```python
from build123d import *

# Parameters (mm, degrees)
BOSS_EXTRUDE1_DEPTH             = 3
BOSS_EXTRUDE2_START             = -6
BOSS_EXTRUDE2_DEPTH             = 6
TAP_DRILL_FOR_M3X0_5_TAP1_D     = 2.5
TAP_DRILL_FOR_M3X0_5_TAP1_DEPTH = 10
TAP_DRILL_FOR_M3X0_5_TAP1_TIP   = 0.751075774
M3_CLEARANCE_HOLE1_D            = 3.4
M3_CLEARANCE_HOLE1_DEPTH        = 10
M3_CLEARANCE_HOLE1_TIP          = 1.021463052
M3_CLEARANCE_HOLE2_D            = 3.4
M3_CLEARANCE_HOLE2_DEPTH        = 10
M3_CLEARANCE_HOLE2_TIP          = 1.021463052
BOSS_EXTRUDE3_START             = 2.5
SKETCH9_R                       = 1.7
BOSS_EXTRUDE3_DEPTH             = 2.5
TAP_DRILL_FOR_M3X0_5_TAP2_D     = 2.5
TAP_DRILL_FOR_M3X0_5_TAP2_DEPTH = 10
TAP_DRILL_FOR_M3X0_5_TAP2_TIP   = 0.751075774
SKETCH8_W                       = 1.5
SKETCH8_H                       = 3.5
CUT_EXTRUDE1_DEPTH              = 15
FILLET3_R                       = 3
FILLET4_R                       = 10


# Some blends are built 0.0001 mm under size
with BuildPart() as part:
    # Sketch1 → Boss-Extrude1 (new body)
    with BuildSketch(Plane.XY):
        with BuildLine():
            Line((-5.729559867, 10.267386408), (-20.186344056, -8.782393513))
            ThreePointArc((-20.186344056, -8.782393513), (-19.418100816, -14.386838385), (-13.813655944, -13.618595145))
            Line((-13.813655944, -13.618595145), (0, 4.583731333))
            Line((0, 4.583731333), (13.813655944, -13.618595145))
            ThreePointArc((13.813655944, -13.618595145), (19.418100816, -14.386838385), (20.186344056, -8.782393513))
            Line((20.186344056, -8.782393513), (5.729559867, 10.267386408))
            Line((5.729559867, 10.267386408), (19.254422206, 19.495329447))
            ThreePointArc((19.254422206, 19.495329447), (20.822087446, 23.979186794), (17, 26.799505671))
            Line((17, 26.799505671), (7, 26.799505671))
            Line((7, 26.799505671), (7, 66.799505671))
            ThreePointArc((7, 66.799505671), (0, 73.799505671), (-7, 66.799505671))
            Line((-7, 66.799505671), (-7, 26.799505671))
            Line((-7, 26.799505671), (-17, 26.799505671))
            ThreePointArc((-17, 26.799505671), (-20.822087446, 23.979186794), (-19.254422206, 19.495329447))
            Line((-19.254422206, 19.495329447), (-5.729559867, 10.267386408))
        make_face()
    extrude(amount=BOSS_EXTRUDE1_DEPTH)

    # Sketch1<3> → Boss-Extrude2 (add)
    with BuildSketch(Plane.XY.offset(BOSS_EXTRUDE2_START)):
        with BuildLine():
            ThreePointArc((-21, 22.799505671), (-20.536784473, 20.931042241), (-19.254422206, 19.495329447))
            ThreePointArc((-19.254422206, 19.495329447), (-15.13153657, 19.262721197), (-13, 22.799505671))
            ThreePointArc((-13, 22.799505671), (-13.463215527, 24.667969101), (-14.745577794, 26.103681895))
            ThreePointArc((-14.745577794, 26.103681895), (-15.820318877, 26.621593117), (-17, 26.799505671))
            ThreePointArc((-17, 26.799505671), (-19.828427125, 25.627932795), (-21, 22.799505671))
        make_face()
        with BuildLine():
            ThreePointArc((14.745577794, 26.103681895), (13.695823776, 20.545083465), (19.254422206, 19.495329447))
            ThreePointArc((19.254422206, 19.495329447), (20.536784473, 20.931042241), (21, 22.799505671))
            ThreePointArc((21, 22.799505671), (19.828427125, 25.627932795), (17, 26.799505671))
            ThreePointArc((17, 26.799505671), (15.820318877, 26.621593117), (14.745577794, 26.103681895))
        make_face()
        with BuildLine():
            ThreePointArc((20.186344056, -8.782393513), (14.581899184, -8.014150273), (13.813655944, -13.618595145))
            ThreePointArc((13.813655944, -13.618595145), (15.221293063, -14.783258853), (17, -15.200494329))
            ThreePointArc((17, -15.200494329), (19.828427125, -14.028921454), (21, -11.200494329))
            ThreePointArc((21, -11.200494329), (20.791132827, -9.924832976), (20.186344056, -8.782393513))
        make_face()
        with BuildLine():
            ThreePointArc((-17, -15.200494329), (-15.221293063, -14.783258853), (-13.813655944, -13.618595145))
            ThreePointArc((-13.813655944, -13.618595145), (-13.208867173, -12.476155682), (-13, -11.200494329))
            ThreePointArc((-13, -11.200494329), (-15.724338647, -7.409361502), (-20.186344056, -8.782393513))
            ThreePointArc((-20.186344056, -8.782393513), (-20.791132827, -9.924832976), (-21, -11.200494329))
            ThreePointArc((-21, -11.200494329), (-19.828427125, -14.028921454), (-17, -15.200494329))
        make_face()
    extrude(amount=BOSS_EXTRUDE2_DEPTH)

    # Tap Drill for M3x0.5 Tap1
    with Locations(Plane(origin=(0, 0, -6), x_dir=(-1, 0, 0), z_dir=(0, 0, -1))):
        with Locations((17, 22.799505671), (-17, 22.799505671)):
            Hole(TAP_DRILL_FOR_M3X0_5_TAP1_D / 2, depth=TAP_DRILL_FOR_M3X0_5_TAP1_DEPTH)
            with Locations((0, 0, -(TAP_DRILL_FOR_M3X0_5_TAP1_DEPTH + TAP_DRILL_FOR_M3X0_5_TAP1_TIP / 2))):  # 118° drill point
                Cone(0, TAP_DRILL_FOR_M3X0_5_TAP1_D / 2, TAP_DRILL_FOR_M3X0_5_TAP1_TIP, mode=Mode.SUBTRACT)

    # M3 Clearance Hole1
    with Locations(Plane(origin=(0, 0, -6), x_dir=(-1, 0, 0), z_dir=(0, 0, -1))):
        with Locations((-17, -11.200494329), (17, -11.200494329)):
            Hole(M3_CLEARANCE_HOLE1_D / 2, depth=M3_CLEARANCE_HOLE1_DEPTH)
            with Locations((0, 0, -(M3_CLEARANCE_HOLE1_DEPTH + M3_CLEARANCE_HOLE1_TIP / 2))):  # 118° drill point
                Cone(0, M3_CLEARANCE_HOLE1_D / 2, M3_CLEARANCE_HOLE1_TIP, mode=Mode.SUBTRACT)

    # M3 Clearance Hole2
    with Locations(Plane.XY.offset(3)):
        with Locations((0, 11.200494329)):
            Hole(M3_CLEARANCE_HOLE2_D / 2, depth=M3_CLEARANCE_HOLE2_DEPTH)
            with Locations((0, 0, -(M3_CLEARANCE_HOLE2_DEPTH + M3_CLEARANCE_HOLE2_TIP / 2))):  # 118° drill point
                Cone(0, M3_CLEARANCE_HOLE2_D / 2, M3_CLEARANCE_HOLE2_TIP, mode=Mode.SUBTRACT)

    # Sketch9 → Boss-Extrude3 (add)
    with BuildSketch(Plane(origin=(0, 0, 0), x_dir=(-1, 0, 0), z_dir=(0, 0, -1)).offset(BOSS_EXTRUDE3_START)):
        with BuildLine():
            Line((7, 66.799505671), (4.365625, 66.799505671))
            Line((4.365625, 66.799505671), (4.365625, 26.799505671))
            Line((4.365625, 26.799505671), (-4.365625, 26.799505671))
            Line((-4.365625, 26.799505671), (-4.365625, 66.799505671))
            Line((-4.365625, 66.799505671), (-7, 66.799505671))
            Line((-7, 66.799505671), (-7, 26.799505671))
            Line((-7, 26.799505671), (-17, 26.799505671))
            ThreePointArc((-17, 26.799505671), (-13.177912554, 21.619824548), (-19.254422206, 19.495329447))
            Line((-19.254422206, 19.495329447), (-5.729559867, 10.267386408))
            Line((-5.729559867, 10.267386408), (-20.186344056, -8.782393513))
            ThreePointArc((-20.186344056, -8.782393513), (-14.581899184, -8.014150273), (-13.813655944, -13.618595145))
            Line((-13.813655944, -13.618595145), (0, 4.583731333))
            Line((0, 4.583731333), (13.813655944, -13.618595145))
            ThreePointArc((13.813655944, -13.618595145), (14.581899184, -8.014150273), (20.186344056, -8.782393513))
            Line((20.186344056, -8.782393513), (5.729559867, 10.267386408))
            Line((5.729559867, 10.267386408), (19.254422206, 19.495329447))
            ThreePointArc((19.254422206, 19.495329447), (13.177912554, 21.619824548), (17, 26.799505671))
            Line((17, 26.799505671), (7, 26.799505671))
            Line((7, 26.799505671), (7, 66.799505671))
        make_face()
        with Locations(Location((0, 11.200494329, 0), (0, 0, 179.999999992))):
            Circle(SKETCH9_R, mode=Mode.SUBTRACT)
    extrude(amount=-BOSS_EXTRUDE3_DEPTH)

    # Tap Drill for M3x0.5 Tap2
    with Locations(Plane(origin=(0, 0, 0), x_dir=(-1, 0, 0), z_dir=(0, 0, -1))):
        with Locations((0, 30.58245731), (0, 47.72934455)):
            Hole(TAP_DRILL_FOR_M3X0_5_TAP2_D / 2, depth=TAP_DRILL_FOR_M3X0_5_TAP2_DEPTH)
            with Locations((0, 0, -(TAP_DRILL_FOR_M3X0_5_TAP2_DEPTH + TAP_DRILL_FOR_M3X0_5_TAP2_TIP / 2))):  # 118° drill point
                Cone(0, TAP_DRILL_FOR_M3X0_5_TAP2_D / 2, TAP_DRILL_FOR_M3X0_5_TAP2_TIP, mode=Mode.SUBTRACT)

    # Sketch8 → Cut-Extrude1 (cut)
    with BuildSketch(Plane.XY.offset(3)):
        with Locations((5, 42.72934455)):
            Rectangle(SKETCH8_W, SKETCH8_H)
        with Locations((-5, 42.72934455)):
            Rectangle(SKETCH8_W, SKETCH8_H)
        with Locations((5, 52.72934455)):
            Rectangle(SKETCH8_W, SKETCH8_H)
        with Locations((-5, 52.72934455)):
            Rectangle(SKETCH8_W, SKETCH8_H)
        with Locations((-5, 62.72934455)):
            Rectangle(SKETCH8_W, SKETCH8_H)
        with Locations((5, 62.72934455)):
            Rectangle(SKETCH8_W, SKETCH8_H)
    extrude(amount=-CUT_EXTRUDE1_DEPTH, mode=Mode.SUBTRACT)

    # Fillet3
    # the kernel refuses this fillet: 3 mm, written as the material it adds along each edge
    with BuildSketch(Plane(origin=(4.365625, 66.799505671, 0), x_dir=(0, 0, -1), z_dir=(1, 0, 0))) as fillet3_piece_1_section:
        with BuildLine():
            CenterArc((3, 2.958039892), FILLET3_R, 180, 80.405931773)
            Line((0, 2.958039892), (0, 0))
            Line((0, 0), (2.5, 0))
        make_face()
    fillet3_piece_1 = extrude(amount=10.029474729, mode=Mode.PRIVATE)
    fillet3_piece_1 = fillet3_piece_1 & Plane(origin=(0, 66.799505671, -0.704129577), x_dir=(1, 0, 0), z_dir=(0, 0, -1)) * Cylinder(7, 32, mode=Mode.PRIVATE)
    add(fillet3_piece_1)
    with BuildSketch(Plane(origin=(-14.395099729, 66.799505671, 0), x_dir=(0, 0, -1), z_dir=(1, 0, 0))) as fillet3_piece_2_section:
        with BuildLine():
            CenterArc((3, 2.958039892), FILLET3_R, 180, 80.405931773)
            Line((0, 2.958039892), (0, 0))
            Line((0, 0), (2.5, 0))
        make_face()
    fillet3_piece_2 = extrude(amount=10.029474729, mode=Mode.PRIVATE)
    fillet3_piece_2 = fillet3_piece_2 & Plane(origin=(0, 66.799505671, -0.704129577), x_dir=(1, 0, 0), z_dir=(0, 0, -1)) * Cylinder(7, 32, mode=Mode.PRIVATE)
    add(fillet3_piece_2)

    # Fillet4
    fillet4_edges = [part.edges().sort_by_distance(p)[0] for p in [
        (7, 26.799505671, 0.25),
        (-7, 26.799505671, 0.25),
    ]]
    fillet(fillet4_edges, radius=FILLET4_R - 0.0001)  # a hair under: the kernel refuses the full size


solid = part.part
```
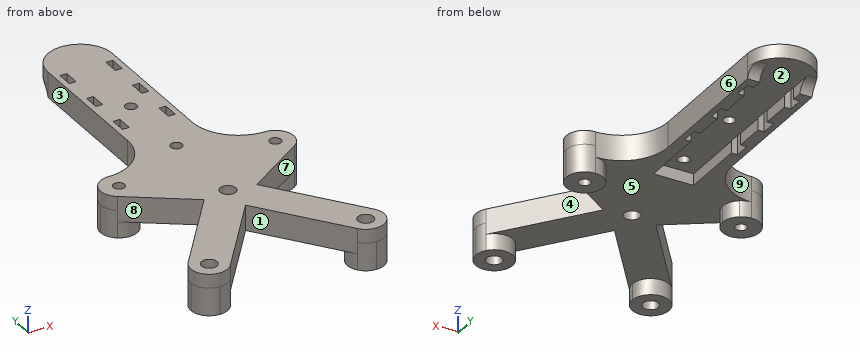
Check sheet for the modelled part. Datum: model origin and axes. Units: mm. Face numbers are marked on the shaded views. A direction names the side the tool comes from. Give positions to 0.01 mm unless a question says otherwise; leave off trailing zeros. Write each loop counter-clockwise with the first axis right and the second up, starting at its lowest first coordinate (ties: lowest second). Pieces come first, ordered by that corner, then holes. Notation, with made-up numbers: (-24, 89) -> (-13, 89) arc R13 cw to (-13, 114) -> close; hole circle Ø8 at (34.25, -35.75). An arc over 180 degrees is marked (long way). Use CSV: the item, a comma, the result in double quotes. Start each with the question number.
Q1. Cross-section at D-D on y = -4.5. Enter the section's corners in (x, z).
Q2. Tool access check on the marked faces 5, 6, 7, 8 and 9. Record the directions out of +Z, -Z, +X, -X, +Y, -Y that give a thin tool (end or side, any length) a straight path to the whole face; none if there is none.
Q3. Release check for a two-part mould opening along X. For the marked faces 1, 2, 3 and 4 record: +X half, -X half, draft (parallel to the pull), parting line (faces both ways), or undercut.
Q4. Scan lines: line 1 along X through (y, z) = (42.5, 2.5); line 2 along Y through (x, z) = (17, 0.5); line 3 along X through (y, z) = (46.5, -0.5). Record each from-to range of solid material in increasing order.
Q5. Cross-section at C-C on y = 39.5. Enter the section's corners in (x, z), and give its area (3 significant figures).
Q6. Depth check by flat-ended pin: P1, Ø0.9, axis at y = 42.5, z = 2, coming from the +X side; P2, Ø1.2, axis at x = 5.5, z = 0.5, coming from the -Y side; P3, Ø5, axis at x = 3, y = 31.5, coming from the -Z side. Enter the tip coordinate at first touch or a pass-through.
Q7. Cross-section at B-B on x = -9. Enter the section's corners in (y, z), and give its area (3 significant figures).
Q8. Cross-section at A-A on z = -4. Enter the section's corners in (x, y).
Working result:
1,outline,"(-16.94, -2.5) -> (-6.89, -2.5) -> (-6.89, 3) -> (-16.94, 3) -> close; (6.89, -2.5) -> (16.94, -2.5) -> (16.94, 3) -> (6.89, 3) -> close"
2,face 5,"-Z"
2,face 6,"+Z, -Z, +X, +Y"
2,face 7,"+Z, -Z, +X"
2,face 8,"+Z, -Z, -X"
2,face 9,"+Z, -Z, -X, +Y"
3,face 1,"undercut"
3,face 2,"undercut"
3,face 3,"-X half"
3,face 4,"+X half"
4,line 1,"x = -7 to -5.75, -4.25 to 4.25, 5.75 to 7"
4,line 2,"y = -15.2 to -12.9, -9.5 to -4.58, 17.96 to 21.55, 24.05 to 26.8"
4,line 3,"x = -7 to -4.37, 4.37 to 7"
5,outline,"(-7, -2.5) -> (-4.37, -2.5) -> (-4.37, 0) -> (4.37, 0) -> (4.37, -2.5) -> (7, -2.5) -> (7, 3) -> (-7, 3) -> close"
5,area,"55.2 mm^2"
6,P1,"stops at x = 7"
6,P2,"stops at y = -3.45"
6,P3,"stops at z = -2.5"
7,outline,"(-7.28, -2.5) -> (5.96, -2.5) -> (5.96, 3) -> (-7.28, 3) -> close; (12.5, -2.5) -> (30.8, -2.5) -> (30.8, 3) -> (12.5, 3) -> close"
7,area,"173 mm^2"
8,outline,"circle Ø8 at (-17, -11.2); circle Ø8 at (-17, 22.8); circle Ø8 at (17, -11.2); circle Ø8 at (17, 22.8); hole circle Ø3.4 at (-17, -11.2); hole circle Ø2.5 at (-17, 22.8); hole circle Ø3.4 at (17, -11.2); hole circle Ø2.5 at (17, 22.8)"
